The listing builds one solid part. Answer for the finished solid, in the listing's coordinates (mm). Face numbers are marked on the shaded views. A direction names the side the tool comes from. Round coordinates to 2 decimals unless told otherwise and drop trailing zeros. Loops run counter-clockwise (first coordinate to the right, second up) from the corner with the lowest first, then second, coordinate; pieces in that order, holes last. Notation, with made-up numbers: (-38.5, 70.25) - (-10.5, 70.25) arc R31 ccw to (-10.5, 94.25) - close; hole circle Ø3 at (50, 49). An arc over 180 degrees is marked (long way). Write item = value, one per line. Start each with the question number.
1) Section D-D, the plane x = 5 is taken. Determine the outline of the cut face in (y, z), and give its area (3 significant figures).
2) Section B-B, the plane z = 3 is taken. Determine the outline of the cut face in (x, y), and give its area (3 significant figures).
3) Section C-C, the plane z = 32 is taken. Determine the outline of the cut face in (x, y), and give its area (3 significant figures).
4) A tool of negligible diameter and unlimited length cuts with its end or side. For the marked faces 1 and 2, from which of +Z, -Z, +X, -X, +Y, -Y can it reach the whole face along a straight path? Write none if from no direction.
5) Section A-A, the plane x = 0 is taken. Determine the outline of the cut face in (y, z).
6) Straight lines are drawn through the part: line 1 along Z through (x, y) = (-3.75, 5.5); line 2 along X through (y, z) = (-0.25, 2.5); line 3 along X through (y, z) = (-3.25, 14.5). For each, find the intervals that lie inside material, in ascending order.
7) Given pin 1 Ø5 at (y, z) = (0, 18) entering from -X; pin 2 Ø2 at (y, z) = (4, 14.5) entering from -X; pin 3 Ø4 at (x, z) = (-3, 30.5) entering from -Y, each flat-ended and moving along its own axis, determine where each tip first touches the part or whether it passes through.
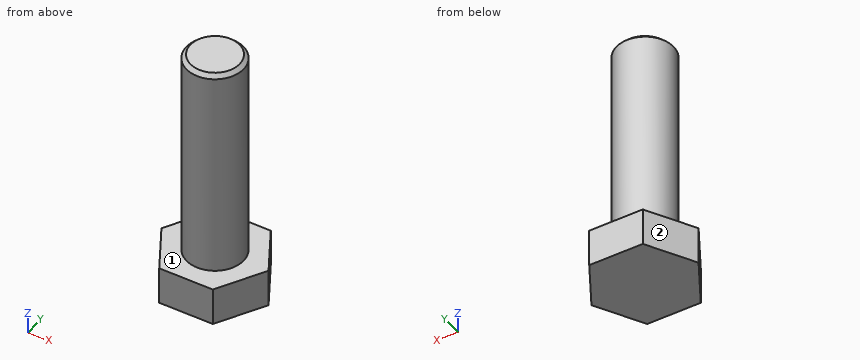
from build123d import *

# Parameters (mm, degrees)
EXTRUDE_1_DEPTH = 5.3
SKETCH_2_R      = 4
EXTRUDE_2_DEPTH = 30
CHAMFER_1_SIZE  = 0.5545


with BuildPart() as part:
    # Эскиз1 → Бобышка-Вытянуть1 (new body)
    with BuildSketch(Plane.XY):
        Polygon((3.75277675, 6.5), (-3.75277675, 6.5), (-7.505553499, 0), (-3.75277675, -6.5), (3.75277675, -6.5), (7.505553499, 0), align=None)
    extrude(amount=EXTRUDE_1_DEPTH)

    # Эскиз2 → Бобышка-Вытянуть2 (add)
    with BuildSketch(Plane.XY.offset(5.3)):
        Circle(SKETCH_2_R)
    extrude(amount=EXTRUDE_2_DEPTH)

    # Фаска1
    chamfer_1_edges = [part.edges().sort_by_distance(p)[0] for p in [
        (-4, 0, 35.3),
    ]]
    chamfer(chamfer_1_edges, length=CHAMFER_1_SIZE)


solid = part.part
Geometry check:
q1.outline = (-4.34, 0) - (4.34, 0) - (4.34, 5.3) - (-4.34, 5.3) - close
q1.area = 46.0 mm2
q2.outline = (-7.51, 0) - (-3.75, -6.5) - (3.75, -6.5) - (7.51, 0) - (3.75, 6.5) - (-3.75, 6.5) - close
q2.area = 146 mm2
q3.outline = circle Ø8 at (0, 0)
q3.area = 50.3 mm2
q4.face_1 = +Z
q4.face_2 = +Z, -Z, -X, +Y
q5.outline = (-6.5, 0) - (6.5, 0) - (6.5, 5.3) - (4, 5.3) - (4, 34.75) - (3.45, 35.3) - (-3.45, 35.3) - (-4, 34.75) - (-4, 5.3) - (-6.5, 5.3) - close
q6.line_1 = 0 to 5.3
q6.line_2 = -7.36 to 7.36
q6.line_3 = -2.33 to 2.33
q7.pin_1 = -4
q7.pin_2 = -2.65
q7.pin_3 = -3.87
